```python
from build123d import *

# Parameters (mm, degrees)
SKETCH1_R           = 2.7051
BOSS_EXTRUDE1_DEPTH = 2.032
CUT_EXTRUDE1_DEPTH  = 90.633545506
BOSS_EXTRUDE2_START = -2.54
SKETCH2_3_R         = 4.7625
BOSS_EXTRUDE2_DEPTH = 2.54
BOSS_EXTRUDE3_START = -71.12
SKETCH2_4_R         = 4.7625
BOSS_EXTRUDE3_DEPTH = 2.54
SKETCH3_W           = 2.54
SKETCH3_H           = 63.5
CUT_EXTRUDE2_DEPTH  = 74.9775539
FILLET1_R           = 2.54
FILLET2_R           = 2.54
FILLET3_R           = 2.54
BOSS_EXTRUDE4_START = 1.27
SKETCH4_R           = 5.842
SKETCH4_R_2         = 4.7625
BOSS_EXTRUDE4_DEPTH = 1.27
FILLET4_R           = 1.27
SKETCH5_R           = 5.842
SKETCH5_R_2         = 4.7625
BOSS_EXTRUDE5_DEPTH = 1.27
FILLET5_R           = 1.27
SKETCH6_R           = 3.937
CUT_EXTRUDE3_DEPTH  = 2.54


with BuildPart() as part:
    # Sketch1 → Boss-Extrude1 (new body)
    with BuildSketch(Plane(origin=(0, 0, 0), x_dir=(1, 0, 0), z_dir=(0, 1, 0))):
        Polygon((-38.1, -47.1551), (-20.32, -47.1551), (20.32, -47.1551), (38.1, -47.1551), (38.1, 16.3449), (-38.1, 16.3449), align=None)
        with Locations(Location((-20.32, 0, 0), (0, 0, 270))):
            Circle(SKETCH1_R, mode=Mode.SUBTRACT)
        with Locations(Location((20.32, 0, 0), (0, 0, 270))):
            Circle(SKETCH1_R, mode=Mode.SUBTRACT)
    extrude(amount=BOSS_EXTRUDE1_DEPTH)

    # Sketch2 → Cut-Extrude1 (cut, through all)
    with BuildSketch(Plane(origin=(38.1, 0, 0), x_dir=(0, 0, -1), z_dir=(1, 0, 0))):
        Polygon((-47.1551, 2.032), (-47.1551, 0), (-45.909587262, 0), align=None)
    extrude(amount=-CUT_EXTRUDE1_DEPTH, mode=Mode.SUBTRACT)

    # Sketch2<3> → Boss-Extrude2 (add)
    with BuildSketch(Plane(origin=(38.1, 0, 0), x_dir=(0, 0, -1), z_dir=(1, 0, 0)).offset(BOSS_EXTRUDE2_START)):
        with BuildLine():
            Line((-17.216664477, 2.032), (-31.930573826, 14.492637507))
            Line((-31.930573826, 14.492637507), (-38.61588269, 25.193525887))
            Line((-38.61588269, 25.193525887), (-39.715274256, 26.953275014))
            ThreePointArc((-39.715274256, 26.953275014), (-51.649026967, 29.426309307), (-56.151659952, 18.101264116))
            Line((-56.151659952, 18.101264116), (-54.398825604, 14.970427636))
            Line((-54.398825604, 14.970427636), (-47.1551, 2.032))
            Line((-47.1551, 2.032), (-24.145873396, 2.032))
            Line((-24.145873396, 2.032), (-17.216664477, 2.032))
        make_face()
        with Locations((-47.1551, 21.082)):
            Circle(SKETCH2_3_R, mode=Mode.SUBTRACT)
    extrude(amount=-BOSS_EXTRUDE2_DEPTH)

    # Sketch2<4> → Boss-Extrude3 (add)
    with BuildSketch(Plane(origin=(38.1, 0, 0), x_dir=(0, 0, -1), z_dir=(1, 0, 0)).offset(BOSS_EXTRUDE3_START)):
        with BuildLine():
            Line((-17.216664477, 2.032), (-31.930573826, 14.492637507))
            Line((-31.930573826, 14.492637507), (-38.61588269, 25.193525887))
            Line((-38.61588269, 25.193525887), (-39.715274256, 26.953275014))
            ThreePointArc((-39.715274256, 26.953275014), (-51.649026967, 29.426309307), (-56.151659952, 18.101264116))
            Line((-56.151659952, 18.101264116), (-54.398825604, 14.970427636))
            Line((-54.398825604, 14.970427636), (-47.1551, 2.032))
            Line((-47.1551, 2.032), (-24.145873396, 2.032))
            Line((-24.145873396, 2.032), (-17.216664477, 2.032))
        make_face()
        with Locations((-47.1551, 21.082)):
            Circle(SKETCH2_4_R, mode=Mode.SUBTRACT)
    extrude(amount=-BOSS_EXTRUDE3_DEPTH)

    # Sketch3 → Cut-Extrude2 (cut, through all)
    with BuildSketch(Plane(origin=(0, 2.032, 0), x_dir=(1, 0, 0), z_dir=(0, 1, 0))):
        with Locations((-36.83, -15.4051)):
            Rectangle(SKETCH3_W, SKETCH3_H)
        Polygon((35.56, -47.1551), (38.1, -47.1551), (38.1, 16.3449), (36.83, 16.3449), (35.56, 16.3449), align=None)
    extrude(amount=-CUT_EXTRUDE2_DEPTH, mode=Mode.SUBTRACT)

    # Fillet1
    fillet1_edges = [part.edges().sort_by_distance(p)[0] for p in [
        (34.29, 2.032, 17.216664477),
        (33.02, 2.032, 32.185882239),
        (-33.02, 2.032, 32.185882239),
        (-34.29, 2.032, 17.216664477),
    ]]
    fillet(fillet1_edges, radius=FILLET1_R)

    # Fillet2
    fillet2_edges = [part.edges().sort_by_distance(p)[0] for p in [
        (-35.56, 1.016, -16.3449),
    ]]
    fillet(fillet2_edges, radius=FILLET2_R)

    # Fillet3
    fillet3_edges = [part.edges().sort_by_distance(p)[0] for p in [
        (35.56, 1.016, -16.3449),
    ]]
    fillet(fillet3_edges, radius=FILLET3_R)

    # Sketch4 → Boss-Extrude4 (add)
    with BuildSketch(Plane(origin=(-33.02, 0, 0), x_dir=(0, 0, -1), z_dir=(1, 0, 0)).offset(BOSS_EXTRUDE4_START)):
        with Locations((-47.1551, 21.082)):
            Circle(SKETCH4_R)
        with Locations((-47.1551, 21.082)):
            Circle(SKETCH4_R_2, mode=Mode.SUBTRACT)
    extrude(amount=-BOSS_EXTRUDE4_DEPTH)

    # Fillet4
    fillet4_edges = [part.edges().sort_by_distance(p)[0] for p in [
        (-33.02, 21.082, 52.9971),
    ]]
    fillet(fillet4_edges, radius=FILLET4_R - 0.0001)  # a hair under: the kernel refuses the full size

    # Sketch5 → Boss-Extrude5 (add)
    with BuildSketch(Plane.ZY.offset(-33.02)):
        with Locations(Location((47.1551, 21.082, 0), (0, 0, 180))):
            Circle(SKETCH5_R)
        with Locations(Location((47.1551, 21.082, 0), (0, 0, 180))):
            Circle(SKETCH5_R_2, mode=Mode.SUBTRACT)
    extrude(amount=BOSS_EXTRUDE5_DEPTH)

    # Fillet5
    fillet5_edges = [part.edges().sort_by_distance(p)[0] for p in [
        (33.02, 21.082, 52.9971),
    ]]
    fillet(fillet5_edges, radius=FILLET5_R - 0.0001)  # a hair under: the kernel refuses the full size

    # Sketch6 → Cut-Extrude3 (cut)
    with BuildSketch(Plane(origin=(0, 2.032, 0), x_dir=(1, 0, 0), z_dir=(0, 1, 0))):
        with Locations(Location((-20.32, 0, 0), (0, 0, 270))):
            Circle(SKETCH6_R)
        with Locations(Location((20.32, 0, 0), (0, 0, 270))):
            Circle(SKETCH6_R)
    extrude(amount=-CUT_EXTRUDE3_DEPTH, mode=Mode.SUBTRACT)


solid = part.part
```
Read the model definition and answer for the solid it produces. Units are mm, in the model's axes. A direction names the side the tool comes from. Coordinates: 2 decimals unless noted, no trailing zeros. Write each loop counter-clockwise with the first axis right and the second up, starting at its lowest first coordinate (ties: lowest second). Pieces come first, ordered by that corner, then holes. Notation, with made-up numbers: (54.5, 17) -> (112.5, 17) arc R21 ccw to (112.5, 27) -> close; hole circle Ø2 at (25.25, -10.5). An arc over 180 degrees is marked (long way). Return JSON: item names as keys, results as strings.
1. Each of these flat-tipped pins is pushed along its axis until it touches: P1, Ø7.5, axis at y = 21.08, z = 47.16, coming from the -X side; P2, Ø9, axis at x = 20.32, z = 0, coming from the -Y side. Where does it stop, or does it pass through?
Found:
{"P1": "through", "P2": "y = 0"}
2. A tool of negligible diameter and unlimited length cuts with its end or side. For faces 1 (the face through (-31.75, 16, 46)), 2 (the face through (-33.02, 15, 43)), 3 (the face through (-32.3, 2.8, 32.2)), 4 (the face through (0, 2.032, 15)), 5 (the face through (0.498, 1.002, 46.524)), from which of +Z, -Z, +X, -X, +Y, -Y can it reach the whole face along a straight path? Write none if from no direction.
Found:
{"face 1": "+Z, -Z, +Y", "face 2": "none", "face 3": "+Z, -Z", "face 4": "-Z, +Y", "face 5": "+Z, +X, -X, -Y"}
3. Determine the mould class of faces 6 (the face through (-33.63, 22.51, 42.61)), 7 (the face through (0, 0, 14)), 8 (the face through (-16.417, 1.03, -0.513)) for opening direction Y: pulls with the +Y half, pulls with the -Y half, needs draft (parallel to the pull), parting line crosses it, or undercut.
Found:
{"face 6": "undercut", "face 7": "pulls with the -Y half", "face 8": "needs draft"}
4. Find the intervals of material crossed by line 1 along X through (y, z) = (1.4, 0); line 2 along X through (y, z) = (5.5, 43.5); line 3 along Y through (x, z) = (13.5, 11), in increasing order. Write a range as from..to.
Found:
{"line 1": "-35.56..-24.26, -16.38..16.38, 24.26..35.56", "line 2": "-35.56..-33.02, 33.02..35.56", "line 3": "0..2.03"}
5. A cutting plane is placed at C-C (y = 7). Determine the outline of the cut face in (x, z).
Found:
{"outline": "(-35.56, 23.08) -> (-33.02, 23.08) -> (-33.02, 49.94) -> (-35.56, 49.94) -> close; (33.02, 23.08) -> (35.56, 23.08) -> (35.56, 49.94) -> (33.02, 49.94) -> close"}
6. A cutting plane is placed at A-A (x = 20.32). Determine the outline of the cut face in (y, z), and give its area (3 significant figures).
Found:
{"outline": "(0, -16.34) -> (2.03, -16.34) -> (2.03, -3.94) -> (0, -3.94) -> close; (0, 3.94) -> (2.03, 3.94) -> (2.03, 47.16) -> (0, 45.91) -> close", "area": "112 mm2"}
7. A cutting plane is placed at D-D (z = 23.5). Determine the outline of the cut face in (x, y).
Found:
{"outline": "(-35.56, 0) -> (35.56, 0) -> (35.56, 7.35) -> (33.02, 7.35) -> (33.02, 4.57) arc R2.54 cw to (30.48, 2.03) -> (-30.48, 2.03) arc R2.54 cw to (-33.02, 4.57) -> (-33.02, 7.35) -> (-35.56, 7.35) -> close"}
8. A cutting plane is placed at B-B (z = 0). Determine the outline of the cut face in (x, y), and give its area (3 significant figures).
Found:
{"outline": "(-35.56, 0) -> (-24.26, 0) -> (-24.26, 2.03) -> (-35.56, 2.03) -> close; (-16.38, 0) -> (16.38, 0) -> (16.38, 2.03) -> (-16.38, 2.03) -> close; (24.26, 0) -> (35.56, 0) -> (35.56, 2.03) -> (24.26, 2.03) -> close", "area": "113 mm2"}
